Autodesk Inventor part; units mm, degrees
ref_plane "YZ Plane" through (0, 0, 0) normal (1, 0, 0) x (0, 1, 0)
ref_plane "XZ Plane" through (0, 0, 0) normal (0, 1, 0) x (-1, 0, 0)
ref_plane "XY Plane" through (0, 0, 0) normal (0, 0, 1) x (1, 0, 0)
sketch "Sketch1" plane through (0, 0, 0) normal (1, 0, 0) x (0, 1, 0)
  line L0 (-4.7, -13.5) -> (-8.7, -13.5)
  line L1 (-8.7, -13.5) -> (-8.7, -20.5)
  line L2 (-8.7, -20.5) -> (8.7, -20.5)
  line L3 (8.7, -20.5) -> (8.7, 20.5)
  line L4 (8.7, 20.5) -> (-4.7, 20.5)
  line L5 (-4.7, 20.5) -> (-4.7, 5.5)
  line L6 (-4.7, 5.5) -> (5.7, 5.5)
  line L7 (5.7, 5.5) -> (5.7, -17.5)
  line L8 (5.7, -17.5) -> (-4.7, -17.5)
  line L9 (-4.7, -17.5) -> (-4.7, -13.5)
  line L10 (8.7, 20.5) -> (-8.7, -20.5) construction
  point P0 (0, 0)
  point P1 (0, 0)
  dimension "d0" = 4
  dimension "d1" = 4
  dimension "d2" = 10.4
  dimension "d3" = 3
  dimension "d4" = 3
  dimension "d5" = 23
  dimension "d6" = 10.4
  dimension "d7" = 15
extrude "Outline" add sketch "Sketch1" along normal mid plane 95
sketch "Sketch3" plane through (-47.5, -4.7, 20.5) normal (0, 0, 1) x (1, 0, 0)
  line L0 (0, 0) -> (95, 0)
  line L1 (74.6, 0) -> (33.6, 0)
  line L2 (33.6, 0) -> (33.6, 10.4)
  line L3 (33.6, 10.4) -> (74.6, 10.4)
  line L4 (74.6, 10.4) -> (74.6, 0)
  line L5 (95, 13.4) -> (95, 0)
  line L6 (0, 0) -> (0, 13.4)
  line L7 (0, 10.4) -> (95, 10.4)
  line L8 (95, 0) -> (95, 10.4)
  line L9 (0, 0) -> (95, 0)
  line L10 (0, 10.4) -> (0, 0)
  point P0 (47.5, 4.7)
  point P1 (33.6, 0)
  dimension "d22" = 33.6
  dimension "d26" = 20.4
extrude "DriverCutout" cut sketch "Sketch3" against normal up to next contours L2 L3 L4 L0
sketch "Sketch2" plane through (-47.5, 8.7, 20.5) normal (0, 1, 0) x (1, 0, 0)
  line L0 (0, 15) -> (33.6, 15)
  line L1 (95, 0) -> (95, 15)
  line L2 (0, 0) -> (33.6, 0)
  line L3 (0, 15) -> (0, 0)
  line L4 (74.6, 0) -> (74.6, 15)
  line L5 (74.6, 15) -> (95, 15)
  line L6 (74.6, 0) -> (95, 0)
  line L7 (33.6, 15) -> (33.6, 0)
  line L8 (10, 5) -> (16.8, 10) construction
  line L9 (16.8, 10) -> (23.6, 5) construction
  line L10 (74.6, 0) -> (74.6, 15) construction
  line L11 (23.6, 5) -> (33.6, 5) construction
  line L12 (33.6, 0) -> (33.6, 15) construction
  line L13 (10, 5) -> (0, 5) construction
  line L14 (74.6, 15) -> (95, 0) construction
  point P0 (47.5, 20.5)
  point P1 (84.8, 7.5)
  dimension "d27" = 5
  dimension "d28" = 5
  dimension "d29" = 10
hole "ScrewHoles" at (-37.5, 8.7, 15.5) at (-30.7, 8.7, 10.5) at (-23.9, 8.7, 15.5) at (37.3, 8.7, 13) direction (0, -1, 0) diameter 3.1 depth 13.4 counterbore diameter 6 counterbore depth 9.4
properties part number "Receptacle_V2_3DPrint"
Model file for the job. Use its own axes, mm. A direction names the side the tool comes from. Coordinates: 2 decimals unless noted, no trailing zeros. Write each loop counter-clockwise with the first axis right and the second up, starting at its lowest first coordinate (ties: lowest second). Pieces come first, ordered by that corner, then holes. Notation, with made-up numbers: (82, -31.75) -> (132, -31.75) arc R12 cw to (132, -24.75) -> close; hole circle Ø9 at (59, 31). An arc over 180 degrees is marked (long way). One line per item, written item: value. Start each with the question number.
1) Which spindle directions (+Z, -Z, +X, -X, +Y, -Y) get a long thin tool onto all of the face, cutting with end or side? Do faces 4 (the face through (37, 0, 5.5)), 5 (the face through (35.27, 3.93, 10.79)), 6 (the face through (-1, 5.7, -2)), 7 (the face through (-1, -7, -13.5)). Say none if no direction does.
2) Slice it at B-B on x = -30.7. Write the cut outline in (y, z), then the cut area to 3 significant figures.
3) Slice it at A-A on y = -1.75. Write the cut outline in (x, z), then the cut area to 3 significant figures.
4) Probe probe 1 along Z at (x, y) = (-37.5, -1.6); probe 2 along Z at (x, y) = (-30.7, -2.3); probe 3 along X at (y, z) = (-2.4, 15.5). List the from-to ranges inside material, lowest first.
5) Pull direction Y, two halves, no side cores. Call faces 1 (the face through (-1, 1, -17.5)), 2 (the face through (-1, -8.7, -17)), 3 (the face through (-31, 0, 5.5)): +Y half, -Y half, draft (parallel to the pull), parting line (faces both ways), or undercut.
6) Flat gauge pins, fed straight in: pin 1 Ø3 at (x, z) = (-37.5, 15.5) entering from -Y; pin 2 Ø1.2 at (x, y) = (13, -7.5) entering from +Z; pin 3 Ø9.5 at (x, z) = (-30.7, 10.5) entering from -Y; pin 4 Ø5.5 at (x, z) = (-23.9, 15.5) entering from +Y. Where does each tip first touch, or does it go through?
7) Slice it at D-D on z = 1.5. Write the cut outline in (x, y), then the cut area to 3 significant figures.
8) Slice it at C-C on x = -3. Write the cut outline in (y, z).
Answers follow:
1. face 4: +X, -X, -Y
1. face 5: +Y
1. face 6: none
1. face 7: +Z, +X, -X, -Y
2. outline: (-8.7, -20.5) -> (8.7, -20.5) -> (8.7, 7.5) -> (-0.7, 7.5) -> (-0.7, 8.95) -> (-4.7, 8.95) -> (-4.7, 5.5) -> (5.7, 5.5) -> (5.7, -17.5) -> (-4.7, -17.5) -> (-4.7, -13.5) -> (-8.7, -13.5) -> close; (-4.7, 12.05) -> (-0.7, 12.05) -> (-0.7, 13.5) -> (8.7, 13.5) -> (8.7, 20.5) -> (-4.7, 20.5) -> close
2. area: 269 mm2
3. outline: (-47.5, -20.5) -> (47.5, -20.5) -> (47.5, -17.5) -> (-47.5, -17.5) -> close; (-47.5, 5.5) -> (-13.9, 5.5) -> (-13.9, 20.5) -> (-47.5, 20.5) -> close; (27.1, 5.5) -> (47.5, 5.5) -> (47.5, 20.5) -> (27.1, 20.5) -> close; hole circle Ø3.1 at (-37.5, 15.5); hole circle Ø3.1 at (-30.7, 10.5); hole circle Ø3.1 at (-23.9, 15.5); hole circle Ø3.1 at (37.3, 13)
3. area: 1,060 mm2
4. probe 1: -20.5 to -17.5, 5.5 to 13.95, 17.05 to 20.5
4. probe 2: -20.5 to -17.5, 5.5 to 8.95, 12.05 to 20.5
4. probe 3: -47.5 to -39.05, -35.95 to -25.45, -22.35 to -13.9, 27.1 to 47.5
5. face 1: undercut
5. face 2: -Y half
5. face 3: draft
6. pin 1: through
6. pin 2: z = -13.5
6. pin 3: y = -4.7
6. pin 4: y = -0.7
7. outline: (-47.5, 5.7) -> (47.5, 5.7) -> (47.5, 8.7) -> (-47.5, 8.7) -> close
7. area: 285 mm2
8. outline: (-8.7, -20.5) -> (8.7, -20.5) -> (8.7, 20.5) -> (5.7, 20.5) -> (5.7, -17.5) -> (-4.7, -17.5) -> (-4.7, -13.5) -> (-8.7, -13.5) -> close
